from build123d import *

# Parameters (mm, degrees)
BOSS_EXTRUDE1_DEPTH = 108.204878078
BOSS_EXTRUDE2_DEPTH = 108.204878078
BOSS_EXTRUDE3_DEPTH = 108.204878078


with BuildPart() as part:
    # Sketch3 → Boss-Extrude1 (new body, symmetric)
    with BuildSketch(Plane.XY):
        Polygon((-153.024806093, 0), (0, 153.024806093), (153.024806093, 0), (0, -153.024806093), align=None)
    extrude(amount=BOSS_EXTRUDE1_DEPTH, both=True)

    # Sketch4 → Boss-Extrude2 (add, symmetric)
    with BuildSketch(Plane(origin=(0, 0, 0), x_dir=(1, 0, 0), z_dir=(0, 1, 0))):
        Polygon((-153.024806093, 0), (0, 153.024806093), (153.024806093, 0), (0, -153.024806093), align=None)
    extrude(amount=BOSS_EXTRUDE2_DEPTH, both=True)

    # Sketch5 → Boss-Extrude3 (add, symmetric)
    with BuildSketch(Plane(origin=(0, 0, 0), x_dir=(0, 0, -1), z_dir=(1, 0, 0))):
        Polygon((-153.024806093, 0), (0, 153.024806093), (153.024806093, 0), (0, -153.024806093), align=None)
    extrude(amount=BOSS_EXTRUDE3_DEPTH, both=True)


solid = part.part
Build history of the part. All positions in model axes, mm. A direction names the side the tool comes from. Give positions to 0.01 mm unless a question says otherwise; leave off trailing zeros. Write each loop counter-clockwise with the first axis right and the second up, starting at its lowest first coordinate (ties: lowest second). Pieces come first, ordered by that corner, then holes. Notation, with made-up numbers: (59, -10.5) - (84, -10.5) arc R17 ccw to (84, -2.5) - close; hole circle Ø9 at (79.5, 68). An arc over 180 degrees is marked (long way). Use one line per item in the form item = value. Start each with the question number.
1. Band-saw the part on C-C on y = 85.5. Write the cut outline in (x, z).
2. Drop flat-ended pins along their axis: pin 1 Ø5 at (x, z) = (-50.5, 102) entering from +Y; pin 2 Ø19 at (y, z) = (92, 61) entering from -X; pin 3 Ø8 at (x, y) = (-102.5, 93.5) entering from -Z. Give the stop position or say it passes through.
3. Band-saw the part on A-A on z = 12. Write the cut outline in (x, y).
4. Band-saw the part on B-B on x = -57.5. Write the cut outline in (y, z).
5. Band-saw the part on D-D on z = -85. Write the cut outline in (x, y).
6. 3-axis set-ups, long thin cutter, end or side, ignore diameter. For faces 1 (the face through (108.205, 1, -126)), 2 (the face through (1, -108.205, -126)), 3 (the face through (-76.956, -95.658, -76.069)): which of +Z, -Z, +X, -X, +Y, -Y reach the whole face in a straight line?
7. Probe line 1 (X direction, y = 2.5, z = -128). List the from-to ranges inside material, lowest first. Write a range as [from, to].
Conclusion:
q1.outline = (-153.02, 0) - (-108.2, -44.82) - (-108.2, -67.52) - (-85.5, -67.52) - (-67.52, -85.5) - (-67.52, -108.2) - (-44.82, -108.2) - (0, -153.02) - (44.82, -108.2) - (67.52, -108.2) - (67.52, -85.5) - (85.5, -67.52) - (108.2, -67.52) - (108.2, -44.82) - (153.02, 0) - (108.2, 44.82) - (108.2, 67.52) - (85.5, 67.52) - (67.52, 85.5) - (67.52, 108.2) - (44.82, 108.2) - (0, 153.02) - (-44.82, 108.2) - (-67.52, 108.2) - (-67.52, 85.5) - (-85.5, 67.52) - (-108.2, 67.52) - (-108.2, 44.82) - close
q2.pin_1 = 108.2
q2.pin_2 = -108.2
q2.pin_3 = -63.52
q3.outline = (-153.02, 0) - (-141.02, -12) - (-141.02, -108.2) - (-108.2, -108.2) - (-108.2, -141.02) - (-12, -141.02) - (0, -153.02) - (12, -141.02) - (108.2, -141.02) - (108.2, -108.2) - (141.02, -108.2) - (141.02, -12) - (153.02, 0) - (141.02, 12) - (141.02, 108.2) - (108.2, 108.2) - (108.2, 141.02) - (12, 141.02) - (0, 153.02) - (-12, 141.02) - (-108.2, 141.02) - (-108.2, 108.2) - (-141.02, 108.2) - (-141.02, 12) - close
q4.outline = (-153.02, 0) - (-108.2, -44.82) - (-108.2, -95.52) - (-95.52, -95.52) - (-95.52, -108.2) - (-44.82, -108.2) - (0, -153.02) - (44.82, -108.2) - (95.52, -108.2) - (95.52, -95.52) - (108.2, -95.52) - (108.2, -44.82) - (153.02, 0) - (108.2, 44.82) - (108.2, 95.52) - (95.52, 95.52) - (95.52, 108.2) - (44.82, 108.2) - (0, 153.02) - (-44.82, 108.2) - (-95.52, 108.2) - (-95.52, 95.52) - (-108.2, 95.52) - (-108.2, 44.82) - close
q5.outline = (-153.02, 0) - (-108.2, -44.82) - (-108.2, -68.02) - (-85, -68.02) - (-68.02, -85) - (-68.02, -108.2) - (-44.82, -108.2) - (0, -153.02) - (44.82, -108.2) - (68.02, -108.2) - (68.02, -85) - (85, -68.02) - (108.2, -68.02) - (108.2, -44.82) - (153.02, 0) - (108.2, 44.82) - (108.2, 68.02) - (85, 68.02) - (68.02, 85) - (68.02, 108.2) - (44.82, 108.2) - (0, 153.02) - (-44.82, 108.2) - (-68.02, 108.2) - (-68.02, 85) - (-85, 68.02) - (-108.2, 68.02) - (-108.2, 44.82) - close
q6.face_1 = -Z, +X, +Y, -Y
q6.face_2 = -Z, +X, -X, -Y
q6.face_3 = -Z, -X, -Y
q7.line_1 = [-108.2, 108.2]
